The listing builds one solid part. Answer for the finished solid, in the listing's coordinates (mm). A direction names the side the tool comes from. Give positions to 0.01 mm unless a question says otherwise; leave off trailing zeros. Loops run counter-clockwise (first coordinate to the right, second up) from the corner with the lowest first, then second, coordinate; pieces in that order, holes last. Notation, with made-up numbers: (40.25, 12) -> (61.25, 12) arc R12 ccw to (61.25, 22) -> close; hole circle Ø4 at (73, -25.5). An arc over 180 degrees is marked (long way). One line per question, with ' | ' between items. Start each with the question number.
from build123d import *

# Parameters (mm, degrees)
SKETCH1_W      = 19.05
SKETCH1_H      = 19.05
EXTRUDE1_DEPTH = 4.7752
SKETCH2_R      = 2.1844
SKETCH2_R_2    = 1.5875
EXTRUDE2_DEPTH = 5.7752
SKETCH4_W      = 1.016
SKETCH4_H      = 2.3876
EXTRUDE3_DEPTH = 20.05


with BuildPart() as part:
    # Sketch1 → Extrude1 (new body)
    with BuildSketch(Plane.XY):
        with Locations((-131.857958108, -85.722466515)):
            Rectangle(SKETCH1_W, SKETCH1_H)
    extrude(amount=EXTRUDE1_DEPTH)

    # Sketch2 → Extrude2 (cut, through all)
    with BuildSketch(Plane.XY.offset(4.7752)):
        with Locations((-131.857958108, -85.722466515)):
            Circle(SKETCH2_R)
        with Locations((-125.507958108, -92.072466515)):
            Circle(SKETCH2_R_2)
        with Locations(Location((-138.207958108, -79.372466515, 0), (0, 0, 180))):  # turned: the seam where the file's is
            Circle(SKETCH2_R_2)
    extrude(amount=-EXTRUDE2_DEPTH, mode=Mode.SUBTRACT)

    # Sketch4 → Extrude3 (cut, through all)
    with BuildSketch(Plane.ZY.offset(141.382958108)):
        with Locations((0.508, -85.316066515)):
            Rectangle(SKETCH4_W, SKETCH4_H)
    extrude(amount=-EXTRUDE3_DEPTH, mode=Mode.SUBTRACT)


solid = part.part
1. The part is cut by section B-B (x = -130.75). Write down the section's boundary in (y, z), plus the area to 3 significant figures.
2. Determine the mould class of faces 3 (the flat face through (-122.333, -86, 2)), 4 (the cylindrical face through (-130.85, -87.66, 2.42)), 5 (the flat face through (-137.7, -86.51, 0.5)) for opening direction X: released by +X, released by -X, zero draft, split by the parting line, or undercut.
3. Straight lines are drawn through the part: L1, parallel to Y at x = -136.5, z = 0.7; L2, parallel to Y at x = -138.25, z = 0.8; L3, parallel to Z at x = -137, y = -84.5. For each, find the intervals that lie inside material, in ascending order.
4. Each of these flat-tipped pins is pushed along its axis until it touches: pin 1 Ø1.9 at (x, y) = (-138, -85.5) entering from -Z; pin 2 Ø1.2 at (x, y) = (-127, -86) entering from -Z; pin 3 Ø3 at (x, y) = (-138.21, -79.37) entering from +Z. Where does it stop, or does it pass through?
5. The part is cut by section C-C (x = -135). Write down the section's boundary in (y, z), plus the area to 3 significant figures.
6. The part is cut by section A-A (y = -85.25). Write down the section's boundary in (x, z).
7. For faces 1 (the cylindrical face through (-138.94, -77.964, 2.421)), 2 (the flat face through (-126.1, -86.51, 0.5)), determine the directions among +Z, -Z, +X, -X, +Y, -Y from which every point of the face is accessible in a straight line to the end or side of a thin tool.
8. The part is cut by section D-D (z = 3.95). Write down the section's boundary in (x, y) (1 decimal).
Check sheet entries:
1) outline: (-95.25, 0) -> (-87.61, 0) -> (-87.61, 4.78) -> (-95.25, 4.78) -> close; (-83.84, 0) -> (-76.2, 0) -> (-76.2, 4.78) -> (-83.84, 4.78) -> close | area: 73.0 mm^2
2) face 3: released by +X | face 4: undercut | face 5: zero draft
3) L1: y = -95.25 to -86.51, -84.12 to -76.2 | L2: y = -95.25 to -86.51, -84.12 to -80.96, -77.79 to -76.2 | L3: z = 1.02 to 4.78
4) pin 1: stops at z = 1.02 | pin 2: stops at z = 0 | pin 3: passes through
5) outline: (-95.25, 0) -> (-86.51, 0) -> (-86.51, 1.02) -> (-84.12, 1.02) -> (-84.12, 0) -> (-76.2, 0) -> (-76.2, 4.78) -> (-95.25, 4.78) -> close | area: 88.5 mm^2
6) outline: (-141.38, 1.02) -> (-133.99, 1.02) -> (-133.99, 4.78) -> (-141.38, 4.78) -> close; (-129.73, 1.02) -> (-122.33, 1.02) -> (-122.33, 4.78) -> (-129.73, 4.78) -> close
7) face 1: +Z, -Z | face 2: -Z, +X, -X
8) outline: (-141.4, -95.2) -> (-122.3, -95.2) -> (-122.3, -76.2) -> (-141.4, -76.2) -> close; hole circle Ø3.2 at (-138.2, -79.4); hole circle Ø4.4 at (-131.9, -85.7); hole circle Ø3.2 at (-125.5, -92.1)
